```python
from build123d import *

# Parameters (mm, degrees)
F0_W      = 40
F0_H      = 40
F1_DEPTH  = 40
F2_R      = 5
F3_DEPTH  = 10
F4_R      = 5
F5_DEPTH  = 10
F6_R      = 5
F7_DEPTH  = 10
F8_R      = 5
F9_DEPTH  = 10
F10_R     = 5
F11_DEPTH = 10
F12_R     = 5
F13_DEPTH = 10


with BuildPart() as f1:
    # F0 (on Top) → F1 (new body)
    with BuildSketch(Plane.XY):
        with Locations((20, -20)):
            Rectangle(F0_W, F0_H)
    extrude(amount=F1_DEPTH)

    # F2 (on face) → F3 (cut)
    with BuildSketch(Plane.XY.offset(40)):
        with Locations((20, -20)):
            Circle(F2_R)
    extrude(amount=-F3_DEPTH, mode=Mode.SUBTRACT)

    # F4 (on face) → F5 (cut)
    with BuildSketch(Plane(origin=(0, 0, 0), x_dir=(-1, 0, 0), z_dir=(0, 1, 0))):
        with Locations((-20, 20)):
            Circle(F4_R)
    extrude(amount=-F5_DEPTH, mode=Mode.SUBTRACT)

    # F6 (on face) → F7 (cut)
    with BuildSketch(Plane(origin=(0, 0, 0), x_dir=(1, 0, 0), z_dir=(0, 0, -1))):
        with Locations((20, 20)):
            Circle(F6_R)
    extrude(amount=-F7_DEPTH, mode=Mode.SUBTRACT)

    # F8 (on face) → F9 (cut)
    with BuildSketch(Plane.XZ.offset(40)):
        with Locations((20, 20)):
            Circle(F8_R)
    extrude(amount=-F9_DEPTH, mode=Mode.SUBTRACT)

    # F10 (on face) → F11 (cut)
    with BuildSketch(Plane.YZ.offset(40)):
        with Locations((-20, 20)):
            Circle(F10_R)
    extrude(amount=-F11_DEPTH, mode=Mode.SUBTRACT)

    # F12 (on face) → F13 (cut)
    with BuildSketch(Plane(origin=(0, 0, 0), x_dir=(0, -1, 0), z_dir=(-1, 0, 0))):
        with Locations((20, 20)):
            Circle(F12_R)
    extrude(amount=-F13_DEPTH, mode=Mode.SUBTRACT)


solid = f1.part
```
Source: CAD feature listing. Evaluate the final solid. Frame: model axes, mm. A direction names the side the tool comes from. Give positions to 0.01 mm unless a question says otherwise; leave off trailing zeros. Order: outer loops, then holes, each group sorted by start corner. A loop starts at its lowest first (then second) coordinate and runs counter-clockwise, first axis right, second up.
(1) Contact query for flat-ended pins moving along their axis: P1, Ø11, axis at y = -21, z = 21.5, coming from the -X side; P2, Ø9, axis at x = 20, z = 20, coming from the +Y side; P3, Ø8, axis at y = -20, z = 20, coming from the -X side; P4, Ø3, axis at x = 22.5, y = -20, coming from the +Z side. Output: stop coordinate, or through.
(2) Material intervals for line 1 along Z through (x, y) = (8, -20); line 2 along Y through (x, z) = (20, 2.5); line 3 along Y through (x, z) = (21.5, 6.5), sorted ascending.
(3) Section query D-D (y = -33.5). Return the cut outline in (x, z).
(4) Section query B-B (x = 20). Return the cut outline in (y, z), plus the area to 3 significant figures.
(5) Section query A-A (z = 32.5). Return the cut outline in (x, y), plus the area to 3 significant figures.
(6) Section query C-C (z = 23). Return the cut outline in (x, y).
(7) Pull-direction query (Z, two-part tool) for faces 6 (the face through (4.93, -18.92, 15.12)), 7 (the face through (18.92, -15.12, 4.93)), 8 (the face through (24, -15, 0)); classes: +Z half, -Z half, draft (parallel to the pull), parting line (faces both ways), or undercut.
(8) Access query for faces 1 (the face through (21.08, -4.93, 15.12)), 2 (the face through (30, -20, 20)), 3 (the face through (20, -30, 20)), 4 (the face through (20, -20, 30)), 5 (the face through (20, -20, 10)). Directions: +Z, -Z, +X, -X, +Y, -Y. A direction counts if a zero-diameter tool reaches every point of the face in a straight line with its end or side. Return the directions, or none.
Outcome:
1. P1: stops at x = 0
1. P2: stops at y = -10
1. P3: stops at x = 10
1. P4: stops at z = 30
2. line 1: z = 0 to 15, 25 to 40
2. line 2: y = -40 to -25, -15 to 0
2. line 3: y = -40 to -24.77, -15.23 to 0
3. outline: (0, 0) - (40, 0) - (40, 40) - (0, 40) - close; hole circle Ø10 at (20, 20)
4. outline: (-40, 0) - (-25, 0) - (-25, 10) - (-15, 10) - (-15, 0) - (0, 0) - (0, 15) - (-10, 15) - (-10, 25) - (0, 25) - (0, 40) - (-15, 40) - (-15, 30) - (-25, 30) - (-25, 40) - (-40, 40) - (-40, 25) - (-30, 25) - (-30, 15) - (-40, 15) - close
4. area: 1,200 mm2
5. outline: (0, -40) - (40, -40) - (40, 0) - (0, 0) - close; hole circle Ø10 at (20, -20)
5. area: 1,520 mm2
6. outline: (0, -40) - (16, -40) - (16, -30) - (24, -30) - (24, -40) - (40, -40) - (40, -24) - (30, -24) - (30, -16) - (40, -16) - (40, 0) - (24, 0) - (24, -10) - (16, -10) - (16, 0) - (0, 0) - (0, -16) - (10, -16) - (10, -24) - (0, -24) - close
7. face 6: undercut
7. face 7: draft
7. face 8: -Z half
8. face 1: +Y
8. face 2: +X
8. face 3: -Y
8. face 4: +Z
8. face 5: -Z
